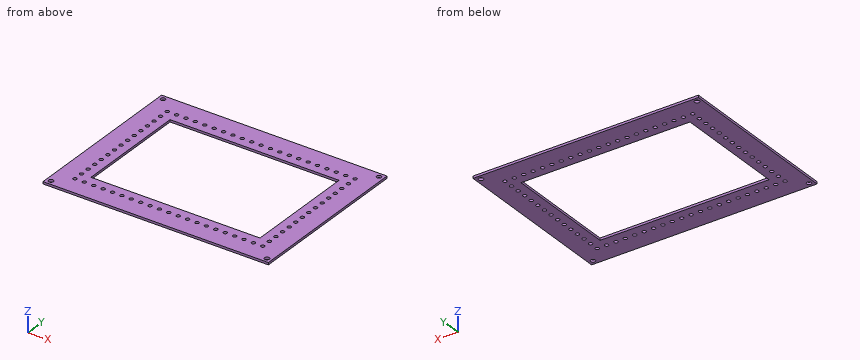
Autodesk Inventor part; units mm, degrees
ref_plane "YZ Plane" through (0, 0, 0) normal (1, 0, 0) x (0, 1, 0)
ref_plane "XZ Plane" through (0, 0, 0) normal (0, 1, 0) x (-1, 0, 0)
ref_plane "XY Plane" through (0, 0, 0) normal (0, 0, 1) x (1, 0, 0)
sketch "Sketch1" plane through (0, 0, 0) normal (0, 0, 1) x (1, 0, 0)
  line L0 (0, 0) -> (228.6, 0)
  line L1 (228.6, 0) -> (228.6, 152.4)
  line L2 (228.6, 152.4) -> (0, 152.4)
  line L3 (0, 152.4) -> (0, 0)
  line L4 (-38.1, -38.1) -> (266.7, -38.1)
  line L5 (266.7, -38.1) -> (266.7, 190.5)
  line L6 (266.7, 190.5) -> (-38.1, 190.5)
  line L7 (-38.1, 190.5) -> (-38.1, -38.1)
  dimension "d0" = 228.6
  dimension "d1" = 152.4
  dimension "d2" = 38.1
extrude "Plate1" add sketch "Sketch1" along normal blind 3.048
sketch "Sketch2" plane through (0, 0, 3.048) normal (0, 0, 1) x (1, 0, 0)
  circle A0 centre (-12.7, -12.7) radius 2.5019
  line L0 (-38.1, -38.1) -> (-38.1, 190.5)
  line L1 (228.6, 0) -> (0, 0)
  line L2 (0, 0) -> (0, 152.4)
  circle A1 centre (0, -12.7) radius 2.5019
  circle A2 centre (12.7, -12.7) radius 2.5019
  circle A3 centre (25.4, -12.7) radius 2.5019
  circle A4 centre (38.1, -12.7) radius 2.5019
  circle A5 centre (50.8, -12.7) radius 2.5019
  circle A6 centre (63.5, -12.7) radius 2.5019
  circle A7 centre (76.2, -12.7) radius 2.5019
  circle A8 centre (88.9, -12.7) radius 2.5019
  circle A9 centre (101.6, -12.7) radius 2.5019
  circle A10 centre (114.3, -12.7) radius 2.5019
  circle A11 centre (127, -12.7) radius 2.5019
  circle A12 centre (139.7, -12.7) radius 2.5019
  circle A13 centre (152.4, -12.7) radius 2.5019
  circle A14 centre (165.1, -12.7) radius 2.5019
  circle A15 centre (177.8, -12.7) radius 2.5019
  circle A16 centre (190.5, -12.7) radius 2.5019
  circle A17 centre (203.2, -12.7) radius 2.5019
  circle A18 centre (215.9, -12.7) radius 2.5019
  circle A19 centre (241.3, -12.7) radius 2.5019
  circle A20 centre (241.3, 0) radius 2.5019
  circle A21 centre (241.3, 12.7) radius 2.5019
  circle A22 centre (241.3, 25.4) radius 2.5019
  circle A23 centre (241.3, 38.1) radius 2.5019
  circle A24 centre (241.3, 50.8) radius 2.5019
  circle A25 centre (241.3, 63.5) radius 2.5019
  circle A26 centre (241.3, 76.2) radius 2.5019
  circle A27 centre (241.3, 88.9) radius 2.5019
  circle A28 centre (241.3, 101.6) radius 2.5019
  circle A29 centre (241.3, 114.3) radius 2.5019
  circle A30 centre (241.3, 127) radius 2.5019
  circle A31 centre (241.3, 165.1) radius 2.5019
  line L3 (0, 152.4) -> (228.6, 152.4)
  circle A32 centre (241.3, 139.7) radius 2.5019
  circle A33 centre (228.6, 165.1) radius 2.5019
  circle A34 centre (215.9, 165.1) radius 2.5019
  circle A35 centre (203.2, 165.1) radius 2.5019
  circle A36 centre (190.5, 165.1) radius 2.5019
  circle A37 centre (177.8, 165.1) radius 2.5019
  circle A38 centre (165.1, 165.1) radius 2.5019
  circle A39 centre (152.4, 165.1) radius 2.5019
  circle A40 centre (139.7, 165.1) radius 2.5019
  circle A41 centre (127, 165.1) radius 2.5019
  circle A42 centre (114.3, 165.1) radius 2.5019
  circle A43 centre (101.6, 165.1) radius 2.5019
  circle A44 centre (88.9, 165.1) radius 2.5019
  circle A45 centre (76.2, 165.1) radius 2.5019
  circle A46 centre (63.5, 165.1) radius 2.5019
  circle A47 centre (50.8, 165.1) radius 2.5019
  circle A48 centre (38.1, 165.1) radius 2.5019
  circle A49 centre (25.4, 165.1) radius 2.5019
  circle A50 centre (12.7, 165.1) radius 2.5019
  circle A51 centre (-12.7, 165.1) radius 2.5019
  circle A52 centre (-12.7, 152.4) radius 2.5019
  circle A53 centre (-12.7, 139.7) radius 2.5019
  circle A54 centre (-12.7, 127) radius 2.5019
  circle A55 centre (-12.7, 114.3) radius 2.5019
  circle A56 centre (-12.7, 101.6) radius 2.5019
  circle A57 centre (-12.7, 88.9) radius 2.5019
  circle A58 centre (-12.7, 76.2) radius 2.5019
  circle A59 centre (-12.7, 63.5) radius 2.5019
  circle A60 centre (-12.7, 50.8) radius 2.5019
  circle A61 centre (-12.7, 38.1) radius 2.5019
  circle A62 centre (-12.7, 25.4) radius 2.5019
  circle A63 centre (-12.7, 12.7) radius 2.5019
  circle A64 centre (-12.7, 0) radius 2.5019
  circle A65 centre (0, 165.1) radius 2.5019
  circle A66 centre (241.3, 152.4) radius 2.5019
  circle A67 centre (228.6, -12.7) radius 2.5019
  dimension "d4" = 5.0038
  dimension "d6" = 12.7
  dimension "d7" = 12.7
  dimension "d10" = 12.7
  dimension "d17" = 5.0038
  dimension "d18" = 25.4
  dimension "d19" = 12.7
  dimension "d22" = 12.7
  dimension "d27" = 5.0038
  dimension "d30" = 25.4
  dimension "d31" = 12.7
  dimension "d34" = 12.7
  dimension "d39" = 5.0038
  dimension "d40" = 25.4
  dimension "d41" = 12.7
  dimension "d44" = 12.7
extrude "Extrusion1" cut sketch "Sketch2" against normal blind 25.4
sketch "Sketch3" plane through (0, 0, 3.048) normal (0, 0, 1) x (1, 0, 0)
  circle A0 centre (-31.75, -31.75) radius 3.175
  line L0 (-38.1, -38.1) -> (-38.1, 190.5)
  line L1 (266.7, -38.1) -> (-38.1, -38.1)
  circle A1 centre (-31.75, 184.15) radius 3.175
  line L2 (-38.1, 190.5) -> (266.7, 190.5)
  circle A2 centre (260.35, 184.15) radius 3.175
  line L3 (266.7, 190.5) -> (266.7, -38.1)
  circle A3 centre (260.35, -31.75) radius 3.175
  point P0 (0, 0)
  dimension "d49" = 6.35
  dimension "d50" = 6.35
  dimension "d51" = 6.35
  dimension "d52" = 6.35
  dimension "d53" = 6.35
  dimension "d54" = 6.35
  dimension "d55" = 6.35
  dimension "d56" = 6.35
  dimension "d57" = 6.35
  dimension "d58" = 6.35
  dimension "d59" = 6.35
  dimension "d60" = 6.35
extrude "Extrusion2" cut sketch "Sketch3" against normal blind 25.4 contours A0 | A1 | A2 | A3
equation "\"d3\" = Thickness"
equation "\"BendRadius\" = Thickness"
equation "\"BendReliefWidth\" = Thickness"
equation "\"BendReliefDepth\" = 0.5 * Thickness"
equation "\"CornerReliefSize\" = 4 * Thickness"
equation "\"MinimumRemnant\" = 2 * Thickness"
equation "\"TransitionRadius\" = BendRadius"
equation "\"JacobiRadiusSize\" = BendRadius"
equation "\"GapSize\" = Thickness"
properties part number "Middle plate"
The listing builds one solid part. Answer for the finished solid, in the listing's coordinates (mm). Coordinates: 2 decimals unless noted, no trailing zeros. Write each loop counter-clockwise with the first axis right and the second up, starting at its lowest first coordinate (ties: lowest second). Pieces come first, ordered by that corner, then holes. Notation, with made-up numbers: (17, 0.5) -> (57, 0.5) arc R18 ccw to (57, 21.5) -> close; hole circle Ø10 at (71.5, 83.5). An arc over 180 degrees is marked (long way). One line per question, with ' | ' between items.
1. Given pin 1 Ø6 at (x, y) = (241.3, 139.7) entering from +Z, flat-ended and moving along its own axis, determine where the tip first touches the part or whether it passes through.
Verdict:
pin 1: stops at z = 3.05
2. Section C-C (z = 0.6) is taken. State how many separate pieces and enclosed holes the cut face has, and give its area (3 significant figures).
Verdict:
separate pieces: 1 | enclosed holes: 73 | area: 33,400 mm^2
3. Section A-A (x = 96) is taken. Determine the outline of the cut face in (y, z).
Verdict:
outline: (-38.1, 0) -> (0, 0) -> (0, 3.05) -> (-38.1, 3.05) -> close; (152.4, 0) -> (190.5, 0) -> (190.5, 3.05) -> (152.4, 3.05) -> close
4. Section B-B (y = 82.5) is taken. Determine the outline of the cut face in (x, z).
Verdict:
outline: (-38.1, 0) -> (0, 0) -> (0, 3.05) -> (-38.1, 3.05) -> close; (228.6, 0) -> (266.7, 0) -> (266.7, 3.05) -> (228.6, 3.05) -> close
5. Straight lines are drawn through the part: line 1 (Y direction, x = 203.2, z = 1.55); line 2 (X direction, y = 42, z = 1.7); line 3 (Y direction, x = 79, z = 0.4). For each, find the intervals that lie inside material, in ascending order.
Verdict:
line 1: y = -38.1 to -15.2, -10.2 to 0, 152.4 to 162.6, 167.6 to 190.5 | line 2: x = -38.1 to 0, 228.6 to 266.7 | line 3: y = -38.1 to 0, 152.4 to 190.5
